Autodesk Inventor part; units mm, degrees
ref_plane "YZ Plane" through (0, 0, 0) normal (1, 0, 0) x (0, 1, 0)
ref_plane "XZ Plane" through (0, 0, 0) normal (0, 1, 0) x (-1, 0, 0)
ref_plane "XY Plane" through (0, 0, 0) normal (0, 0, 1) x (1, 0, 0)
sketch "Sketch1" plane through (0, 0, 0) normal (0, 0, 1) x (1, 0, 0)
  line L0 (-19, 10) -> (19, 10)
  line L1 (19, 10) -> (19, -10)
  line L2 (19, -10) -> (-19, -10)
  line L3 (-19, -10) -> (-19, 10)
  line L4 (-19, 0) -> (19, 0) construction
  line L5 (-13.5, 0) -> (-10, 0) construction
  line L6 (-13.5, -2.75) -> (-10, -2.75)
  line L7 (-10, 2.75) -> (-13.5, 2.75)
  arc A0 (-13.5, 2.75) -> (-13.5, -2.75) centre (-13.5, 0) ccw
  arc A1 (-10, -2.75) -> (-10, 2.75) centre (-10, 0) ccw
  line L8 (0, 10) -> (0, -10) construction
  line L9 (13.5, 0) -> (10, 0) construction
  line L10 (13.5, -2.75) -> (10, -2.75)
  line L11 (10, 2.75) -> (13.5, 2.75)
  arc A2 (13.5, -2.75) -> (13.5, 2.75) centre (13.5, 0) ccw
  arc A3 (10, 2.75) -> (10, -2.75) centre (10, 0) ccw
  point P0 (0, 0)
  point P1 (-11.75, 0)
  point P2 (11.75, 0)
  dimension "d0" = 20
  dimension "d1" = 38
  dimension "d2" = 5.5
  dimension "d3" = 3.5
  dimension "d4" = 10
  dimension "d15" = 23.5
extrude "Extrusion1" add sketch "Sketch1" along normal blind 3
sketch "Sketch2" plane through (0, 0, 3) normal (0, 0, 1) x (1, 0, 0)
  line L0 (19, -10) -> (19, 10)
  line L1 (-19, -10) -> (19, -10)
  line L2 (19, -10) -> (19, -7)
  line L3 (19, -7) -> (-19, -7)
  line L4 (-19, -7) -> (-19, -10)
  point P0 (0, 0)
  dimension "d7" = 3
extrude "Extrusion2" add sketch "Sketch2" along normal blind 17
sketch "Sketch3" plane through (-19, -7, 3) normal (0, 1, 0) x (1, 0, 0)
  line L0 (0, 0) -> (0, -17)
  line L1 (38, -17) -> (0, -17)
  line L2 (38, 0) -> (38, -17)
  line L3 (0, -12) -> (38, -12) construction
  line L4 (4.5, -12) -> (10, -12) construction
  line L5 (4.5, -14.75) -> (10, -14.75)
  line L6 (10, -9.25) -> (4.5, -9.25)
  arc A0 (4.5, -9.25) -> (4.5, -14.75) centre (4.5, -12) ccw
  arc A1 (10, -14.75) -> (10, -9.25) centre (10, -12) ccw
  line L7 (0, 0) -> (38, 0)
  line L8 (19, 0) -> (19, -17) construction
  line L9 (33.5, -12) -> (28, -12) construction
  line L10 (33.5, -14.75) -> (28, -14.75)
  line L11 (28, -9.25) -> (33.5, -9.25)
  arc A2 (33.5, -14.75) -> (33.5, -9.25) centre (33.5, -12) ccw
  arc A3 (28, -9.25) -> (28, -14.75) centre (28, -12) ccw
  point P0 (19, 3)
  point P1 (7.25, -12)
  point P2 (19, -12)
  point P3 (30.75, -12)
  dimension "d10" = 5.5
  dimension "d11" = 5.5
  dimension "d12" = 5
  dimension "d16" = 23.5
extrude "Extrusion3" cut sketch "Sketch3" against normal up to surface (3 mm away) contours A0 L6 A1 L5 | L10 A3 L11 A2
properties part number "L bracket double"
Geometry check sheet. Reference: the model listing, model coordinates, mm. A direction names the side the tool comes from. Coordinates: 2 decimals unless noted, no trailing zeros. Order: outer loops, then holes, each group sorted by start corner. A loop starts at its lowest first (then second) coordinate and runs counter-clockwise, first axis right, second up. Notation, with made-up numbers: (15.25, -25.75) - (52.25, -25.75) arc R22 ccw to (52.25, 9.25) - close; hole circle Ø6 at (45, 73.25). An arc over 180 degrees is marked (long way). Answer in a Markdown table with one row per item. Add a question column.
1) Release check for a two-part mould opening along Z. For faces 5 (the cylindrical face through (6.25, -8.48, 14.94)), 6 (the flat face through (-12, -8, 17.75)), 7 (the flat face through (19, -4.4, 2.5)), 8 (the flat face through (0, 2, 3)) record: +Z half, -Z half, draft (parallel to the pull), parting line (faces both ways), or undercut.
2) Material ranges on line 1 along Z through (x, y) = (-12.5, -8.5); line 2 along Y through (x, z) = (6, 15.75); line 3 along Z through (x, y) = (2, 1.5), recorded low to high. Write a range as [from, to].
3) Set-up check for faces 1 (the cylindrical face through (16.25, 0.06, 1.48)), 2 (the flat face through (0, -10, 10)), 3 (the flat face through (-12, -8, 12.25)), 4 (the flat face through (0, -7, 11)): record each of +Z, -Z, +X, -X, +Y, -Y from which the full face is reachable in a straight line by a thin tool's end or side.
4) Cross-section at C-C, the plane z = 10.5. Record the cut outline in (x, y).
5) Cross-section at D-D, the plane x = 0. Record the cut outline in (y, z).
6) Cross-section at A-A, the plane z = 15. Record the cut outline in (x, y), then the cut area to 3 significant figures.
7) Cross-section at B-B, the plane x = -10.5. Record the cut outline in (y, z).
8) Gauge pin test, flat end, axial feed: P1, Ø4, axis at x = -0.5, z = 17.5, coming from the +Y side. Record the tip position at first contact, or that the pin passes through.
Check result:
| question | item | result |
|---|---|---|
| 1 | face 5 | undercut |
| 1 | face 6 | undercut |
| 1 | face 7 | draft |
| 1 | face 8 | +Z half |
| 2 | line 1 | z = [0, 12.25], [17.75, 20] |
| 2 | line 2 | y = [-10, -7] |
| 2 | line 3 | z = [0, 3] |
| 3 | face 1 | +Z, -Z |
| 3 | face 2 | +Z, -Z, +X, -X, -Y |
| 3 | face 3 | +Y, -Y |
| 3 | face 4 | +Z, +X, -X, +Y |
| 4 | outline | (-19, -10) - (19, -10) - (19, -7) - (-19, -7) - close |
| 5 | outline | (-10, 0) - (10, 0) - (10, 3) - (-7, 3) - (-7, 20) - (-10, 20) - close |
| 6 | outline | (-19, -10) - (-17.25, -10) - (-17.25, -7) - (-19, -7) - close; (-6.25, -10) - (6.25, -10) - (6.25, -7) - (-6.25, -7) - close; (17.25, -10) - (19, -10) - (19, -7) - (17.25, -7) - close |
| 6 | area | 48.0 mm² |
| 7 | outline | (-10, 0) - (-2.75, 0) - (-2.75, 3) - (-7, 3) - (-7, 12.25) - (-10, 12.25) - close; (-10, 17.75) - (-7, 17.75) - (-7, 20) - (-10, 20) - close; (2.75, 0) - (10, 0) - (10, 3) - (2.75, 3) - close |
| 8 | P1 | stops at y = -7 |
